from build123d import *

# Parameters (mm, degrees)
BOSS_EXTRU_1_DEPTH       = 320
BOSS_EXTRU_1_DEPTH_BACK  = 10
ENL_V_MAT_EXTRU_1_DEPTH  = 300
ESQUISSE3_W              = 196.156872589
ESQUISSE3_H              = 6
BOSS_EXTRU_2_DEPTH       = 56.1
ESQUISSE41_W             = 200.156872589
ESQUISSE41_H             = 330
BOSS_EXTRU_9_DEPTH       = 3
ENL_V_MAT_EXTRU_22_DEPTH = 6
CONG_8_R                 = 10
CONG_7_R                 = 0.2
ESQUISSE43_W             = 6.98
ESQUISSE43_H             = 5
BOSS_EXTRU_10_DEPTH      = 0.05
ESQUISSE44_W             = 6
ESQUISSE44_H             = 6
BOSS_EXTRU_11_DEPTH      = 0.05
ESQUISSE45_W             = 6.978514333
ESQUISSE45_H             = 6
BOSS_EXTRU_12_DEPTH      = 0.05
ESQUISSE46_W             = 6
ESQUISSE46_H             = 6
BOSS_EXTRU_13_DEPTH      = 0.05
ENL_V_MAT_EXTRU_23_DEPTH = 3.5
CONG_11_R                = 2.5
ESQUISSE48_W             = 3
ESQUISSE48_H             = 3


with BuildPart() as part:
    # Esquisse1 → Boss.-Extru.1 (new body, two sides)
    with BuildSketch(Plane.XY) as boss_extru_1_sk:
        with BuildLine():
            Line((-107.913003101, 2), (82.243869488, 2))
            ThreePointArc((82.243869488, 2), (84.365189832, 2.878679656), (85.243869488, 5))
            Line((85.243869488, 5), (85.243869488, 17))
            ThreePointArc((85.243869488, 17), (86.708335582, 20.535533906), (90.243869488, 22))
            Line((90.243869488, 22), (116.243869488, 22))
            Line((116.243869488, 22), (121.243869488, 22))
            Line((121.243869488, 22), (121.243869488, 20))
            Line((121.243869488, 20), (116.243869488, 20))
            Line((116.243869488, 20), (90.243869488, 20))
            ThreePointArc((90.243869488, 20), (88.122549145, 19.121320344), (87.243869488, 17))
            Line((87.243869488, 17), (87.243869488, 0))
            Line((87.243869488, 0), (-112.913003101, 0))
            Line((-112.913003101, 0), (-112.913003101, 17))
            ThreePointArc((-112.913003101, 17), (-113.791682758, 19.121320344), (-115.913003101, 20))
            Line((-115.913003101, 20), (-137.913003101, 20))
            Line((-137.913003101, 20), (-142.913003101, 20))
            Line((-142.913003101, 20), (-142.913003101, 22))
            Line((-142.913003101, 22), (-137.913003101, 22))
            Line((-137.913003101, 22), (-115.913003101, 22))
            ThreePointArc((-115.913003101, 22), (-112.377469195, 20.535533906), (-110.913003101, 17))
            Line((-110.913003101, 17), (-110.913003101, 5))
            ThreePointArc((-110.913003101, 5), (-110.034323445, 2.878679656), (-107.913003101, 2))
        make_face()
    extrude(amount=BOSS_EXTRU_1_DEPTH)
    extrude(boss_extru_1_sk.sketch, amount=-BOSS_EXTRU_1_DEPTH_BACK)

    # Esquisse2 → Enlèv. mat.-Extru.1 (cut)
    with BuildSketch(Plane.XZ.offset(-20)):
        with BuildLine():
            Line((-139.784323445, 22.121320344), (-136.284323445, 25.621320344))
            ThreePointArc((-136.284323445, 25.621320344), (-132.041682758, 25.621320344), (-132.041682758, 21.378679656))
            Line((-132.041682758, 21.378679656), (-135.541682758, 17.878679656))
            ThreePointArc((-135.541682758, 17.878679656), (-139.784323445, 17.878679656), (-139.784323445, 22.121320344))
        make_face()
        with BuildLine():
            Line((-136.284323445, 284.378679656), (-139.784323445, 287.878679656))
            ThreePointArc((-139.784323445, 287.878679656), (-139.784323445, 292.121320344), (-135.541682758, 292.121320344))
            Line((-135.541682758, 292.121320344), (-132.041682758, 288.621320344))
            ThreePointArc((-132.041682758, 288.621320344), (-132.041682758, 284.378679656), (-136.284323445, 284.378679656))
        make_face()
        with BuildLine():
            Line((118.115189832, 287.878679656), (114.615189832, 284.378679656))
            ThreePointArc((114.615189832, 284.378679656), (110.372549145, 284.378679656), (110.372549145, 288.621320344))
            Line((110.372549145, 288.621320344), (113.872549145, 292.121320344))
            ThreePointArc((113.872549145, 292.121320344), (118.115189832, 292.121320344), (118.115189832, 287.878679656))
        make_face()
        with BuildLine():
            Line((114.615189832, 25.621320344), (118.115189832, 22.121320344))
            ThreePointArc((118.115189832, 22.121320344), (118.115189832, 17.878679656), (113.872549145, 17.878679656))
            Line((113.872549145, 17.878679656), (110.372549145, 21.378679656))
            ThreePointArc((110.372549145, 21.378679656), (110.372549145, 25.621320344), (114.615189832, 25.621320344))
        make_face()
        with BuildLine():
            Line((116.243869488, 155.403419264), (111.243869488, 155.403419264))
            ThreePointArc((111.243869488, 155.403419264), (108.243869488, 158.403419264), (111.243869488, 161.403419264))
            Line((111.243869488, 161.403419264), (116.243869488, 161.403419264))
            ThreePointArc((116.243869488, 161.403419264), (119.243869488, 158.403419264), (116.243869488, 155.403419264))
        make_face()
        with BuildLine():
            Line((-138.413003101, 161.403419264), (-133.413003101, 161.403419264))
            ThreePointArc((-133.413003101, 161.403419264), (-130.413003101, 158.403419264), (-133.413003101, 155.403419264))
            Line((-133.413003101, 155.403419264), (-138.413003101, 155.403419264))
            ThreePointArc((-138.413003101, 155.403419264), (-141.413003101, 158.403419264), (-138.413003101, 161.403419264))
        make_face()
    extrude(amount=-ENL_V_MAT_EXTRU_1_DEPTH, mode=Mode.SUBTRACT)

    # Esquisse3 → Boss.-Extru.2 (add)
    with BuildSketch(Plane(origin=(0, 0, 0), x_dir=(-1, 0, 0), z_dir=(0, -1, 0))):
        with Locations((12.834566806, -317)):
            Rectangle(ESQUISSE3_W, ESQUISSE3_H)
    extrude(amount=BOSS_EXTRU_2_DEPTH)

    # Esquisse41 → Boss.-Extru.9 (add)
    with BuildSketch(Plane.XZ):
        with Locations((-12.834566806, 155)):
            Rectangle(ESQUISSE41_W, ESQUISSE41_H)
        with BuildLine():
            Line((81.243869488, 314), (-106.913003101, 314))
            Line((-106.913003101, 314), (-106.913003101, 6))
            ThreePointArc((-106.913003101, 6), (-103.984070913, -1.071067812), (-96.913003101, -4))
            Line((-96.913003101, -4), (71.243869488, -4))
            ThreePointArc((71.243869488, -4), (78.3149373, -1.071067812), (81.243869488, 6))
            Line((81.243869488, 6), (81.243869488, 314))
        make_face(mode=Mode.SUBTRACT)
    extrude(amount=BOSS_EXTRU_9_DEPTH)

    # Esquisse24 → Enlèv. mat.-Extru.22 (cut)
    with BuildSketch(Plane.XY.offset(320)):
        Polygon((80.263869488, -3), (69.213869488, -65.686319951), (85.243869488, -65.686319951), (85.243869488, -3), align=None)
        Polygon((-105.934488768, -3), (-94.881199239, -65.686319951), (-110.913003101, -65.686319951), (-110.913003101, -3), align=None)
    extrude(amount=-ENL_V_MAT_EXTRU_22_DEPTH, mode=Mode.SUBTRACT)

    # Congé8
    cong_8_edges = [part.edges().sort_by_distance(p)[0] for p in [
        (-96.571526093, -56.1, 317),
        (70.903693289, -56.1, 317),
    ]]
    fillet(cong_8_edges, radius=CONG_8_R)

    # Congé7
    cong_7_edges = [part.edges().sort_by_distance(p)[0] for p in [
        (-142.913003101, 21, -10),
    ]]
    fillet(cong_7_edges, radius=CONG_7_R)

    # Esquisse43 → Boss.-Extru.10 (add)
    with BuildSketch(Plane.XZ.offset(3)):
        with Locations((83.753869488, 317.5)):
            Rectangle(ESQUISSE43_W, ESQUISSE43_H)
    extrude(amount=BOSS_EXTRU_10_DEPTH)

    # Esquisse44 → Boss.-Extru.11 (add)
    with BuildSketch(Plane(origin=(78.357901362, -13.812500251, 0), x_dir=(0, 0, -1), z_dir=(0.984816589, -0.173598057, 0))):
        with Locations((-317, 7.973810121)):
            Rectangle(ESQUISSE44_W, ESQUISSE44_H)
    extrude(amount=BOSS_EXTRU_11_DEPTH)

    # Esquisse45 → Boss.-Extru.12 (add)
    with BuildSketch(Plane.XZ.offset(3)):
        with Locations((-109.423745935, 317)):
            Rectangle(ESQUISSE45_W, ESQUISSE45_H)
    extrude(amount=BOSS_EXTRU_12_DEPTH)

    # Esquisse46 → Boss.-Extru.13 (add)
    with BuildSketch(Plane(origin=(-103.25320329, -18.206325585, 0), x_dir=(0, 0, 1), z_dir=(-0.984807753, -0.173648178, 0))):
        with Locations((317, 12.440907668)):
            Rectangle(ESQUISSE46_W, ESQUISSE46_H)
    extrude(amount=BOSS_EXTRU_13_DEPTH)

    # Enlèvement de matière-Balayage1: sweep along a path in Esquisse47
    with BuildLine(Plane.XZ.offset(3)) as enl_vement_de_mati_re_balayage1_path:
        Line((84.243869488, 298.46050791), (84.243869488, 5))
        ThreePointArc((84.243869488, 5), (80.729150862, -3.485281374), (72.243869488, -7))
        Line((72.243869488, -7), (-97.913003101, -7))
        ThreePointArc((-97.913003101, -7), (-106.398284476, -3.485281374), (-109.913003101, 5))
        Line((-109.913003101, 5), (-109.913003101, 298.46050791))
    # Esquisse3D1 → Enlèvement de matière-Balayage1 (sweep, cut)
    with BuildSketch(Plane(origin=(-48.798071116, -0.937456497, -5.5), x_dir=(0, -0.624695048, -0.780868809), z_dir=(1, 0, 0))):
        Polygon((0, 0), (1.499268114, -1.874085143), (3.841874542, 0), (2.342606428, 1.874085143), align=None)
    sweep(path=enl_vement_de_mati_re_balayage1_path.line, mode=Mode.SUBTRACT)

    # Esquisse50 → Enlèv. mat.-Extru.23 (cut)
    with BuildSketch(Plane(origin=(0, 0, 314), x_dir=(-1, 0, 0), z_dir=(0, 0, -1))):
        with BuildLine():
            Line((87.39220148, -52.1), (-61.673120332, -52.1))
            ThreePointArc((-61.673120332, -52.1), (-66.172770053, -50.462196601), (-68.566836458, -46.315186396))
            Line((-68.566836458, -46.315186396), (-76.731022999, 0))
            Line((-76.731022999, 0), (102.452534593, 0))
            Line((102.452534593, 0), (94.285855751, -46.315537244))
            ThreePointArc((94.285855751, -46.315537244), (91.891714748, -50.462311102), (87.39220148, -52.1))
        make_face()
    extrude(amount=-ENL_V_MAT_EXTRU_23_DEPTH, mode=Mode.SUBTRACT)

    # Congé11
    cong_11_edges = [part.edges().sort_by_distance(p)[0] for p in [
        (-98.369195172, -23.157768622, 317.5),
        (-91.891714748, -50.462311102, 317.5),
        (-12.859540574, -52.1, 317.5),
        (66.172770053, -50.462196601, 317.5),
        (72.648929728, -23.157593198, 317.5),
    ]]
    fillet(cong_11_edges, radius=CONG_11_R)

    # Enlèvement de matière-Balayage2: sweep along a curve in space
    with BuildLine() as enl_vement_de_mati_re_balayage2_path:
        Line((79.221345133, -8.914209531, 317), (72.358298385, -47.836481777, 317))
        ThreePointArc((72.358298385, -47.836481777, 317), (68.938096952, -53.760444431, 317), (62.510220855, -56.1, 317))
        Line((-8.284645145, -56.1, 317), (62.510220855, -56.1, 317))
        Line((-8.284645145, -56.1, 317), (-88.180529781, -56.1, 317))
        ThreePointArc((-98.028607311, -47.836481777, 317), (-94.608405878, -53.760444431, 317), (-88.180529781, -56.1, 317))
        Line((-104.892599702, -8.908846518, 317), (-98.028607311, -47.836481777, 317))
    # Esquisse48 → Enlèvement de matière-Balayage2 (sweep, cut)
    with BuildSketch(Plane(origin=(0, 0, 0), x_dir=(0, 0, -1), z_dir=(1, 0, 0))):
        with Locations((-317, -55.2)):
            Rectangle(ESQUISSE48_W, ESQUISSE48_H)
    sweep(path=enl_vement_de_mati_re_balayage2_path.line, mode=Mode.SUBTRACT)


solid = part.part
Model file for the job. Use its own axes, mm. A direction names the side the tool comes from. Round coordinates to 2 decimals unless told otherwise and drop trailing zeros. Order: outer loops, then holes, each group sorted by start corner. A loop starts at its lowest first (then second) coordinate and runs counter-clockwise, first axis right, second up.
(1) Band-saw the part on A-A (y = 13.5). List the corners of the cut face in (x, z), then the cut area to 3 significant figures.
(2) Pin check, flat tips, straight feed: pin 1 (1.7 mm diameter, centred on y = -2, z = 132, fed in from -X); pin 2 (24 mm diameter, centred on x = 5.5, y = -24, fed in from -Z); pin 3 (3 mm diameter, centred on x = 22, z = 217, fed in from +Y). Stop position of each tip, or through.
(3) Drill centre lines: line 1 (X direction, y = -1.5, z = 278); line 2 (X direction, y = 7, z = 37); line 3 (Z direction, x = 68, y = -38). Where is each one in solid material? Low to high.
(4) Band-saw the part on B-B (x = -62). List the corners of the cut face in (y, z), then the cut area to 3 significant figures.
(5) Band-saw the part on D-D (x = -125.5). List the corners of the cut face in (y, z), then the cut area to 3 significant figures.
(6) 3-axis set-ups, long thin cutter, end or side, ignore diameter. For faces 1 (the face through (87.244, 7, 153)), 2 (the face through (85.244, 11, 157)), 3 (the face through (-1, -24, 320)), 4 (the face through (-112.913, 7, 153)): which of +Z, -Z, +X, -X, +Y, -Y reach the whole face in a straight line?
(7) Pull direction X, two halves, no side cores. Call faces 5 (the face through (-98.426, -22.834, 314.493)), 6 (the face through (-94.533, -53.823, 319.24)), 7 (the face through (69.01, -53.7, 314.74)): released by +X, released by -X, zero draft, split by the parting line, or undercut.
Verdict:
1. outline: (-112.91, -10) - (-110.91, -10) - (-110.91, 320) - (-112.91, 320) - close; (85.24, -10) - (87.24, -10) - (87.24, 320) - (85.24, 320) - close
1. area: 1,320 mm2
2. pin 1: stops at x = -112.91
2. pin 2: stops at z = 317.5
2. pin 3: stops at y = 2
3. line 1: x = -112.91 to -111.41, -108.41 to -106.91, 81.24 to 82.74, 85.74 to 87.24
3. line 2: x = -112.91 to -110.91, 85.24 to 87.24
3. line 3: z = 317.45 to 320
4. outline: (-56.1, 314) - (-52.1, 314) - (-52.1, 315) arc R2.5 cw to (-49.6, 317.5) - (0, 317.5) - (0, -4) - (-3, -4) - (-3, -5.5) - (-0.94, -5.5) - (-0.94, -8.5) - (-3, -8.5) - (-3, -10) - (2, -10) - (2, 320) - (-56.1, 320) - (-56.1, 318.5) - (-53.7, 318.5) - (-53.7, 315.5) - (-56.1, 315.5) - close
4. area: 820 mm2
5. outline: (20, -10) - (22, -10) - (22, 320) - (20, 320) - close
5. area: 660 mm2
6. face 1: +Z, -Z, +X, -Y
6. face 2: +Z, -Z, +Y
6. face 3: +Z, +X, -X, +Y, -Y
6. face 4: +Z, -Z, -X, -Y
7. face 5: undercut
7. face 6: released by -X
7. face 7: released by +X
